The model under review builds one solid part; all positions refer to its coordinate system, in mm. A direction names the side the tool comes from. Round coordinates to 2 decimals unless told otherwise and drop trailing zeros. Write each loop counter-clockwise with the first axis right and the second up, starting at its lowest first coordinate (ties: lowest second). Pieces come first, ordered by that corner, then holes. Notation, with made-up numbers: M 51,13.5 L 106,13.5 A24 cw 106,35.5 Z; hole C 56,-4 d1. An arc over 180 degrees is marked long. Write item = value, one per line. Start each with the question number.
Item 1: Take a section at A-A, the plane z = 29. Give the boundary of the cut face in (x, y).
Item 2: To check wall thickness, follow line 1 along Z through (x, y) = (-8, 4.5); line 2 along Y through (x, z) = (0, 7.5); line 3 along Y through (x, z) = (0, 21). State the ranges of each line that lie inside material, in increasing order.
Item 3: Take a section at D-D, the plane z = 46. Give the boundary of the cut face in (x, y).
Item 4: Take a section at B-B, the plane z = 20.5. Give the boundary of the cut face in (x, y).
Item 5: For pin 1 Ø8 at (x, z) = (-10, 41) entering from -Y; pin 2 Ø2 at (x, y) = (8.5, 13.5) entering from +Z; pin 3 Ø2 at (x, z) = (-6, 28) entering from +Y; pin 4 Ø1.5 at (y, z) = (-12.5, 46) entering from -X, all flat-tipped, find the tip position at first contact; note any pin that passes through.
Item 6: Take a section at C-C, the plane y = 14. Give the boundary of the cut face in (x, z).
Item 7: Tool access review of faces 1 (the flat face through (-9, -2, 7)), 2 (the flat face through (0, 8, 28)), 3 (the cylindrical face through (1.302, -9.915, 29.815)): name each direction out of +Z, -Z, +X, -X, +Y, -Y from which nothing blocks a thin tool from reaching the whole face with its end or side.
Item 8: The part is to be moulded in two halves that separate along Z. For faces 4 (the conical face through (0.264, 1.187, 35.305)), 5 (the flat face through (-7, 4, 22)), 6 (the cylindrical face through (6.96, 4.6, 27.43)), 7 (the cylindrical face through (13.267, -12.165, 2.028)), say which applies: +Z half, -Z half, draft (parallel to the pull), parting line (faces both ways), or undercut.
from build123d import *

# Parameters (mm, degrees)
ENL_V_MAT_EXTRU_1_DEPTH      = 10
ENL_V_MAT_EXTRU_1_DEPTH_BACK = 10


with BuildPart() as part:
    # Esquisse1 → R_volution1 (revolve)
    with BuildSketch(Plane(origin=(0, 0, 0), x_dir=(0, 0, -1), z_dir=(1, 0, 0)), mode=Mode.PRIVATE) as r_volution1_sk:
        Polygon((-70, 0), (-36, 0), (-32, 7), (0, 7), (0, 18), (-4, 18), (-4, 9), (-7, 9), (-7, 10), (-52, 10), (-52, 6), (-70, 6), align=None)
    revolve(r_volution1_sk.sketch.rotate(Axis((0, 0, 0), (0, 0, 1)), 90), axis=Axis((0, 0, 0), (0, 0, 1)))

    # Esquisse2 → Enl_v. mat.-Extru.1 (cut, two sides: drawn at the far end of the back side and taken through both)
    with BuildSketch(Plane(origin=(0, 0, 0), x_dir=(0, 0, -1), z_dir=(1, 0, 0)).offset(-ENL_V_MAT_EXTRU_1_DEPTH_BACK)):
        with BuildLine():
            Line((-16, 10), (-28, 10))
            Line((-28, 10), (-28, 6))
            ThreePointArc((-28, 6), (-27.414213562, 4.585786438), (-26, 4))
            Line((-26, 4), (-18, 4))
            ThreePointArc((-18, 4), (-16.585786438, 4.585786438), (-16, 6))
            Line((-16, 6), (-16, 10))
        make_face()
    extrude(amount=ENL_V_MAT_EXTRU_1_DEPTH + ENL_V_MAT_EXTRU_1_DEPTH_BACK, mode=Mode.SUBTRACT)


solid = part.part
Response values:
q1.outline = C 0,0 d20; hole C 0,0 d14
q2.line_1 = 0 to 4, 7 to 16.68, 27.32 to 52
q2.line_2 = -10 to -7, 7 to 10
q2.line_3 = -10 to -7
q3.outline = C 0,0 d20
q4.outline = M -9.17,4 A10 ccw long 9.17,4 L 5.74,4 A7 cw long -5.74,4 Z
q5.pin_1 = -8
q5.pin_2 = 4
q5.pin_3 = 8.66
q5.pin_4 = through
q6.outline = M -11.31,0 L 11.31,0 L 11.31,4 L -11.31,4 Z
q7.face_1 = none
q7.face_2 = +X, -X, +Y
q7.face_3 = +Z
q8.face_4 = -Z half
q8.face_5 = undercut
q8.face_6 = undercut
q8.face_7 = draft
